Geometry check sheet. Reference: the model listing, model coordinates, mm. A direction names the side the tool comes from. Coordinates: 2 decimals unless noted, no trailing zeros. Loops run counter-clockwise (first coordinate to the right, second up) from the corner with the lowest first, then second, coordinate; pieces in that order, holes last. Notation, with made-up numbers: M 56.25,60 L 103.25,60 A28 ccw 103.25,81 Z; hole C -6,-13 d9. An arc over 180 degrees is marked long. One line per question, with ' | ' between items. Start each with the question number.
from build123d import *

# Parameters (mm, degrees)
F0_W     = 7.5
F0_H     = 7.5
F0_W_2   = 2.5
F0_H_2   = 2.5
F1_DEPTH = 10
F2_R     = 1
F3_R     = 1


with BuildPart() as f1:
    # F0 (on Front) → F1 (new body)
    with BuildSketch(Plane.XZ):
        Polygon((5, -12.5), (-5, -12.5), (-5, -7.5), (-7.5, -7.5), (-7.5, -15), (7.5, -15), (7.5, -7.5), (5, -7.5), align=None)
        Polygon((-15, -7.5), (-7.5, -7.5), (-7.5, -5), (-12.5, -5), (-12.5, 5), (-7.5, 5), (-7.5, 7.5), (-15, 7.5), align=None)
        with Locations((-11.25, -11.25)):
            Rectangle(F0_W, F0_H)
        with Locations((11.25, -11.25)):
            Rectangle(F0_W, F0_H)
        Polygon((7.5, -5), (7.5, -7.5), (15, -7.5), (15, 7.5), (7.5, 7.5), (7.5, 5), (12.5, 5), (12.5, -5), align=None)
        Polygon((-7.5, 7.5), (-5, 7.5), (-5, 12.5), (5, 12.5), (5, 7.5), (7.5, 7.5), (7.5, 15), (-7.5, 15), align=None)
        with Locations((-11.25, 11.25)):
            Rectangle(F0_W, F0_H)
        with Locations((11.25, 11.25)):
            Rectangle(F0_W, F0_H)
        with Locations((-6.25, 6.25)):
            Rectangle(F0_W_2, F0_H_2)
        with Locations((6.25, 6.25)):
            Rectangle(F0_W_2, F0_H_2)
        with Locations((6.25, -6.25)):
            Rectangle(F0_W_2, F0_H_2)
        with Locations((-6.25, -6.25)):
            Rectangle(F0_W_2, F0_H_2)
    extrude(amount=F1_DEPTH)

    # F2
    f2_edges = [f1.edges().sort_by_distance(p)[0] for p in [
        (-5, -5, 5),
        (-5, -5, 12.5),
        (-12.5, -5, 5),
        (5, -5, 12.5),
        (5, -5, 5),
        (12.5, -5, 5),
        (12.5, -5, -5),
        (5, -5, -5),
        (5, -5, -12.5),
        (-5, -5, -12.5),
        (-5, -5, -5),
        (-12.5, -5, -5),
    ]]
    fillet(f2_edges, radius=F2_R)

    # F3
    f3_edges = [f1.edges().sort_by_distance(p)[0] for p in [
        (15, -10, 0),
        (0, -10, 15),
        (-15, -10, 0),
        (0, -10, -15),
        (-8.75, -10, -5),
        (-15, -5, -15),
        (15, -5, -15),
        (15, -5, 15),
        (-15, -5, 15),
    ]]
    fillet(f3_edges, radius=F3_R)


solid = f1.part
1. Sectioned sample at A-A (z = -10.25). Record the cut outline in (x, y).
2. Tool access check on faces 5 (the cylindrical face through (-0.196, -9.715, 14.699)), 6 (the cylindrical face through (12.801, -9.715, -0.056)), 7 (the cylindrical face through (-4.715, -4.563, 12.199)). Record the directions out of +Z, -Z, +X, -X, +Y, -Y that give a thin tool (end or side, any length) a straight path to the whole face; none if there is none.
3. Depth check by flat-ended pin: pin 1 Ø1 at (x, z) = (4.5, -4) entering from +Y. Enter the tip coordinate at first touch or a pass-through.
4. Draft check along Z on faces 1 (the flat face through (0, -4, 15)), 2 (the flat face through (-15, -4, 0)), 3 (the cylindrical face through (5.301, -4.563, -5.285)), 4 (the flat face through (0, -4, 12.5)). Enter one of: +Z half, -Z half, draft (parallel to the pull), parting line (faces both ways), or undercut.
5. Sectioned sample at B-B (x = 11). Record the cut outline in (y, z).
6. Thickness scan on line 1 (Z direction, x = 7.75, y = -0.75); line 2 (X direction, y = -3.25, z = 0). Record the ranges inside material, lowest first.
Result:
1) outline: M -15,-9 A1 ccw -14,-10 L -6,-10 A1 ccw -5,-9 L -5,0 L -15,0 Z; M 5,-9 A1 ccw 6,-10 L 14,-10 A1 ccw 15,-9 L 15,0 L 5,0 Z
2) face 5: +Z, +X, -X, -Y | face 6: -Y | face 7: +Y, -Y
3) pin 1: passes through
4) face 1: +Z half | face 2: draft | face 3: undercut | face 4: undercut
5) outline: M -10,-14 A1 ccw -9,-15 L 0,-15 L 0,-5 L -9,-5 A1 ccw -10,-6 Z; M -10,6 A1 ccw -9,5 L 0,5 L 0,15 L -9,15 A1 ccw -10,14 Z
6) line 1: z = -15 to -5, 5 to 15 | line 2: x = -15 to -12.5, 12.5 to 15
